Verification items for the finished model (mm, model axes). Face numbers are marked on the shaded views. A direction names the side the tool comes from. Coordinates: 2 decimals unless noted, no trailing zeros. Loops run counter-clockwise (first coordinate to the right, second up) from the corner with the lowest first, then second, coordinate; pieces in that order, holes last. Notation, with made-up numbers: (-31.5, 26) -> (-21.5, 26) arc R11 ccw to (-21.5, 37) -> close; hole circle Ø3 at (4, 78). An arc over 180 degrees is marked (long way). Write item = value, one per line.
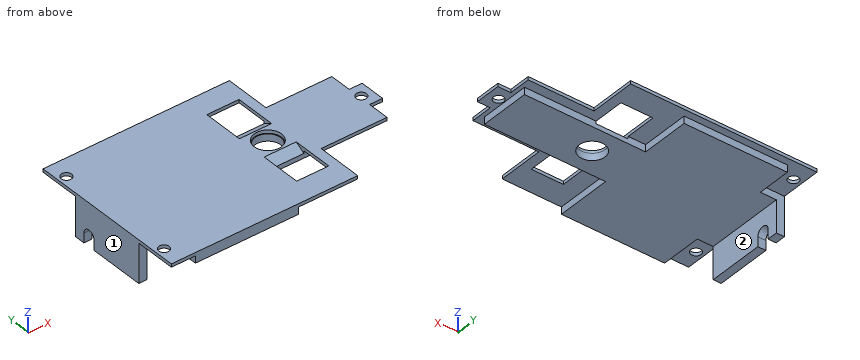
```python
from build123d import *

# Parameters (mm, degrees)
SKETCH4_R           = 1.6
BOSS_EXTRUDE2_DEPTH = 1
BOSS_EXTRUDE3_DEPTH = 2.2
SKETCH6_R           = 4
SKETCH6_W           = 10.008556046
SKETCH6_H           = 9.470821567
CUT_EXTRUDE1_DEPTH  = 57.031418446
CUT_EXTRUDE2_DEPTH  = 10.008556046
SKETCH8_W           = 2.5
SKETCH8_H           = 24.6
BOSS_EXTRUDE4_DEPTH = 10
CUT_EXTRUDE3_REACH  = 89.157
SKETCH10_R          = 4.25
CUT_EXTRUDE4_DEPTH  = 1


with BuildPart() as part:
    # Sketch4 → Boss-Extrude2 (new body)
    with BuildSketch(Plane.XY):
        Polygon((-50.042780229, 25), (8.006844837, 25), (8.006844837, 10.737807635), (28.52438473, 10.737807635), (28.52438473, 3.982032304), (32.555371359, 3.982032304), (32.555371359, -3.982032304), (28.52438473, -3.982032304), (28.52438473, -10.737807635), (8.006844837, -10.737807635), (8.006844837, -25), (-50.042780229, -25), align=None)
        with Locations((-47.542780229, 19)):
            Circle(SKETCH4_R, mode=Mode.SUBTRACT)
        with Locations(Location((-47.542780229, -19, 0), (0, 0, 180))):
            Circle(SKETCH4_R, mode=Mode.SUBTRACT)
        with Locations((29.123529126, 0)):
            Circle(SKETCH4_R, mode=Mode.SUBTRACT)
    extrude(amount=BOSS_EXTRUDE2_DEPTH)

    # Sketch5 → Boss-Extrude3 (add)
    with BuildSketch(Plane(origin=(0, 0, 0), x_dir=(-1, 0, 0), z_dir=(0, 0, -1))):
        Polygon((10.130686795, 7.8), (-27.3, 7.8), (-27.3, -7.8), (10.130686795, -7.8), (10.416393564, -7.8), (10.416393564, -8), (10.416393564, -25), (42.575341492, -25), (42.575341492, -12.3), (50.042780229, -12.3), (50.042780229, 12.3), (42.575341492, 12.3), (42.575341492, 22.8), (10.416393564, 22.8), (10.416393564, 8), (10.416393564, 7.8), align=None)
    extrude(amount=BOSS_EXTRUDE3_DEPTH)

    # Sketch6 → Cut-Extrude1 (cut, through all)
    with BuildSketch(Plane.XY.offset(1)):
        Circle(SKETCH6_R)
        with Locations((0, -12.74225562)):
            Rectangle(SKETCH6_W, SKETCH6_H)
        with Locations((0, 12.74225562)):
            Rectangle(SKETCH6_W, SKETCH6_H)
    extrude(amount=-CUT_EXTRUDE1_DEPTH, mode=Mode.SUBTRACT)

    # Sketch7 → Cut-Extrude2 (cut)
    with BuildSketch(Plane(origin=(-5.004278023, 0, 0), x_dir=(0, 0, -1), z_dir=(1, 0, 0))):
        Polygon((0.904413332, -8.006844837), (-1, -4.814198104), (-1, -8.006844837), (0, -8.006844837), align=None)
    cut_extrude2 = extrude(amount=CUT_EXTRUDE2_DEPTH, mode=Mode.SUBTRACT)

    # Mirror1: Cut-Extrude2 across plane
    add(cut_extrude2.mirror(Plane.ZX), mode=Mode.SUBTRACT)

    # Sketch8 → Boss-Extrude4 (add)
    with BuildSketch(Plane(origin=(0, 0, -2.2), x_dir=(-1, 0, 0), z_dir=(0, 0, -1))):
        with Locations((48.792780229, 0)):
            Rectangle(SKETCH8_W, SKETCH8_H)
    extrude(amount=BOSS_EXTRUDE4_DEPTH)

    # Sketch9 → Cut-Extrude3 (cut, up to next)
    with BuildSketch(Plane.ZY.offset(50.042780229), mode=Mode.PRIVATE) as cut_extrude3_sk1:
        with BuildLine():
            Line((-9.2, 9.061272662), (-12.2, 9.061272662))
            Line((-12.2, 9.061272662), (-12.2, 5.087082771))
            Line((-12.2, 5.087082771), (-9.2, 5.087082771))
            ThreePointArc((-9.2, 5.087082771), (-7.212905055, 7.074177716), (-9.2, 9.061272662))
        make_face()
    cut_extrude3_tool1 = extrude(cut_extrude3_sk1.sketch, amount=-CUT_EXTRUDE3_REACH, mode=Mode.PRIVATE) & part.part
    add(cut_extrude3_tool1.solids().sort_by_distance((-50.04278, 7.074178, -9.898105))[0], mode=Mode.SUBTRACT)

    # Sketch10 → Cut-Extrude4 (cut)
    with BuildSketch(Plane.XY.offset(1)):
        Circle(SKETCH10_R)
    extrude(amount=-CUT_EXTRUDE4_DEPTH, mode=Mode.SUBTRACT)


solid = part.part
```
1) Sectioned sample at C-C, the plane x = 0. Record the cut outline in (y, z).
Ans:
outline = (-25, 0) -> (-17.48, 0) -> (-17.48, 1) -> (-25, 1) -> close; (-7.8, -2.2) -> (-4, -2.2) -> (-4, 0) -> (-4.25, 0) -> (-4.25, 1) -> (-4.81, 1) -> (-7.8, -0.78) -> close; (4, -2.2) -> (7.8, -2.2) -> (7.8, -0.78) -> (4.81, 1) -> (4.25, 1) -> (4.25, 0) -> (4, 0) -> close; (17.48, 0) -> (25, 0) -> (25, 1) -> (17.48, 1) -> close
2) Sectioned sample at D-D, the plane x = 16. Record the cut outline in (y, z), plus the area to 3 significant figures.
Ans:
outline = (-10.74, 0) -> (-7.8, 0) -> (-7.8, -2.2) -> (7.8, -2.2) -> (7.8, 0) -> (10.74, 0) -> (10.74, 1) -> (-10.74, 1) -> close
area = 55.8 mm2
3) Sectioned sample at A-A, the plane y = 19. Record the cut outline in (x, z), plus the area to 3 significant figures.
Ans:
outline = (-50.04, 0) -> (-49.14, 0) -> (-49.14, 1) -> (-50.04, 1) -> close; (-45.94, 0) -> (-42.58, 0) -> (-42.58, -2.2) -> (-10.42, -2.2) -> (-10.42, 0) -> (8.01, 0) -> (8.01, 1) -> (-45.94, 1) -> close
area = 126 mm2
4) Material ranges on line 1 (Y direction, x = -17.5, z = -1.5); line 2 (Z direction, x = -38, y = -11); line 3 (Z direction, x = -43, y = 15.5), recorded low to high.
Ans:
line_1 = -25 to 22.8
line_2 = -2.2 to 1
line_3 = 0 to 1
5) Depth check by flat-ended pin: pin 1 Ø2 at (x, z) = (-46.5, -9) entering from +Y; pin 2 Ø0.5 at (x, z) = (22, 0.5) entering from +Y; pin 3 Ø3.5 at (x, y) = (-47.54, -19) entering from -Z; pin 4 Ø2 at (x, z) = (-48.5, -11) entering from -Y. Enter the tip coordinate at first touch or a pass-through.
Ans:
pin_1 = through
pin_2 = 10.74
pin_3 = 0
pin_4 = -12.3
6) Sectioned sample at B-B, the plane y = 0. Record the cut outline in (x, z).
Ans:
outline = (-50.04, -12.2) -> (-47.54, -12.2) -> (-47.54, -2.2) -> (-4, -2.2) -> (-4, 0) -> (-4.25, 0) -> (-4.25, 1) -> (-50.04, 1) -> close; (4, -2.2) -> (27.3, -2.2) -> (27.3, 0) -> (27.52, 0) -> (27.52, 1) -> (4.25, 1) -> (4.25, 0) -> (4, 0) -> close; (30.72, 0) -> (32.56, 0) -> (32.56, 1) -> (30.72, 1) -> close
7) Tool access check on the marked faces 1 and 2. Record the directions out of +Z, -Z, +X, -X, +Y, -Y that give a thin tool (end or side, any length) a straight path to the whole face; none if there is none.
Ans:
face_1 = +Z, -Z, -X, +Y, -Y
face_2 = -Z, +X, +Y, -Y
